Build history of the part. All positions in model axes, mm. Give positions to 0.01 mm unless a question says otherwise; leave off trailing zeros. Write each loop counter-clockwise with the first axis right and the second up, starting at its lowest first coordinate (ties: lowest second). Pieces come first, ordered by that corner, then holes. Notation, with made-up numbers: M 82.5,2.25 L 138.5,2.25 A9 ccw 138.5,12.25 Z; hole C -15,83 d9. An arc over 180 degrees is marked long. Return JSON: item names as keys, results as strings. Group by question number.
Q1. Band-saw the part on C-C, the plane y = -43. Count the separate pieces of the cut face and the enclosed holes in it, then the cut area to 3 significant figures.
Q2. Band-saw the part on B-B, the plane x = 1.25. Give the cut face in (y, z).
Q3. Band-saw the part on A-A, the plane x = -6.9. Give the cut face in (y, z).
Q4. Wall check: probe 1 along X at (y, z) = (-50.5, -1.5); probe 2 along X at (y, z) = (32, -3); probe 3 along X at (y, z) = (-23, -5.75). Give the ranges that are in metal, low to high.
Q5. Flat gauge pins, fed straight in: pin 1 Ø2 at (x, y) = (1, -24.5) entering from -Z; pin 2 Ø5 at (x, z) = (-6.9, -3) entering from +Y; pin 3 Ø0.6 at (y, z) = (-18, -9) entering from -X. Where does each tip first touch, or does it go through?
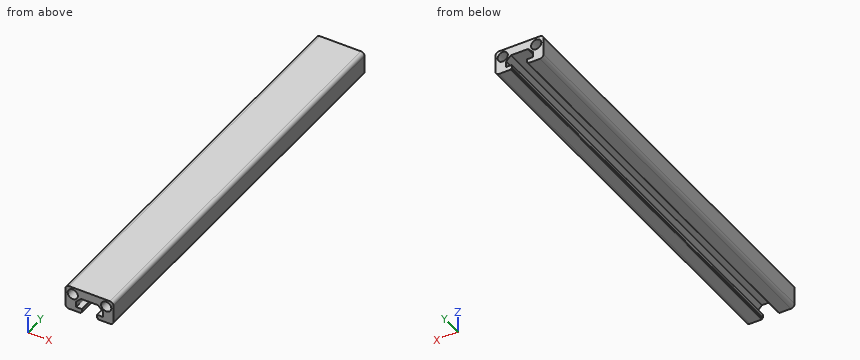
from build123d import *

# Parameters (mm, degrees)
SKETCH_1_R      = 2.1
EXTRUDE_1_DEPTH = 85
FILLET_1_R      = 0.1


with BuildPart() as part:
    # 草图1 → 凸台-拉伸1 (new, symmetric)
    with BuildSketch(Plane(origin=(0, 0, 0), x_dir=(1, 0, 0), z_dir=(0, 1, 0))):
        with BuildLine():
            Line((-3.5, 10), (-3.5, 9.5))
            Line((-3.5, 9.5), (-3.1, 9.5))
            Line((-3.1, 9.5), (-3.1, 8.1))
            Line((-3.1, 8.1), (-5.5, 8.1))
            Line((-5.5, 8.1), (-5.5, 5.701219331))
            Line((-5.5, 5.701219331), (-3.498780669, 3.7))
            Line((-3.498780669, 3.7), (3.498780669, 3.7))
            Line((3.498780669, 3.7), (5.5, 5.701219331))
            Line((5.5, 5.701219331), (5.5, 8.1))
            Line((5.5, 8.1), (3.1, 8.1))
            Line((3.1, 8.1), (3.1, 9.5))
            Line((3.1, 9.5), (3.5, 9.5))
            Line((3.5, 9.5), (3.5, 10))
            Line((3.5, 10), (8.4, 10))
            ThreePointArc((8.4, 10), (9.460660172, 9.560660172), (9.9, 8.5))
            Line((9.9, 8.5), (9.9, 1.5))
            ThreePointArc((9.9, 1.5), (9.460660172, 0.439339828), (8.4, 0))
            Line((8.4, 0), (-8.4, 0))
            ThreePointArc((-8.4, 0), (-9.460660172, 0.439339828), (-9.9, 1.5))
            Line((-9.9, 1.5), (-9.9, 8.5))
            ThreePointArc((-9.9, 8.5), (-9.460660172, 9.560660172), (-8.4, 10))
            Line((-8.4, 10), (-3.5, 10))
        make_face()
        with Locations(Location((-6.9, 3, 0), (0, 0, 270))):
            Circle(SKETCH_1_R, mode=Mode.SUBTRACT)
        with Locations(Location((6.9, 3, 0), (0, 0, 270))):
            Circle(SKETCH_1_R, mode=Mode.SUBTRACT)
    extrude(amount=EXTRUDE_1_DEPTH, both=True)

    # 圆角1
    fillet_1_edges = [part.edges().sort_by_distance(p)[0] for p in [
        (-3.5, 0, -10),
        (-3.5, 0, -9.5),
        (-3.1, 0, -9.5),
        (-3.1, 0, -8.1),
        (-5.5, 0, -8.1),
        (-5.5, 0, -5.701219331),
        (-3.498780669, 0, -3.7),
        (3.498780669, 0, -3.7),
        (5.5, 0, -5.701219331),
        (5.5, 0, -8.1),
        (3.1, 0, -8.1),
        (3.1, 0, -9.5),
        (3.5, 0, -9.5),
        (3.5, 0, -10),
    ]]
    fillet(fillet_1_edges, radius=FILLET_1_R)


solid = part.part
From the geometry:
{
 "1": {"separate pieces": "1", "enclosed holes": "2", "area": "112 mm^2"},
 "2": {"outline": "M -85,-3.7 L 85,-3.7 L 85,0 L -85,0 Z"},
 "3": {"outline": "M -85,-10 L 85,-10 L 85,-5.1 L -85,-5.1 Z; M -85,-0.9 L 85,-0.9 L 85,0 L -85,0 Z"},
 "4": {"probe 1": "x = -9.9 to -8.37, -5.43 to 5.43, 8.37 to 9.9", "probe 2": "x = -9.9 to -9, -4.8 to 4.8, 9 to 9.9", "probe 3": "x = -9.9 to -5.5, 5.5 to 9.9"},
 "5": {"pin 1": "stops at z = -3.7", "pin 2": "stops at y = 85", "pin 3": "stops at x = -9.89"}
}
